Design review of the part built by this model. Coordinates are the model's own, in mm. Face numbers are marked on the shaded views. A direction names the side the tool comes from. Coordinates: 2 decimals unless noted, no trailing zeros. Loops run counter-clockwise (first coordinate to the right, second up) from the corner with the lowest first, then second, coordinate; pieces in that order, holes last. Notation, with made-up numbers: (34, 38) -> (65, 38) arc R23 ccw to (65, 71) -> close; hole circle Ø6 at (52.25, 23.25). An arc over 180 degrees is marked (long way). Answer in a Markdown table with one row per item.
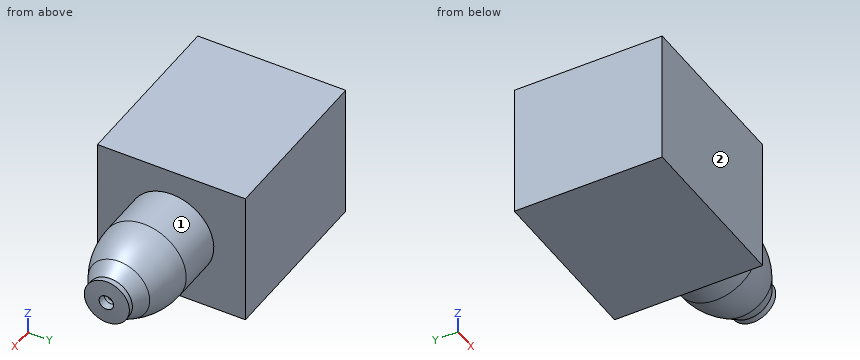
```python
from build123d import *

# Parameters (mm, degrees)
SKETCH1_W           = 52.054588137
SKETCH1_H           = 19.540614726
BOSS_EXTRUDE1_DEPTH = 8.89
SKETCH3_W           = 29.304045921
SKETCH3_H           = 19.540614726
CUT_EXTRUDE1_DEPTH  = 70.835641623


with BuildPart() as part:
    # Model → Revolve1 (revolve)
    with BuildSketch(Plane.XY, mode=Mode.PRIVATE) as revolve1_sk:
        with BuildLine():
            add(Edge.make_bspline(
                [(65.953268304, 2.93538911), (66.613970922, 2.97512211), (66.714344102, 2.980580933)],
                knots=[0.156174428, 0.156174428, 0.156174428, 1, 1, 1], degree=2))
            Line((66.714344102, 2.980580933), (66.8238694, 0.9515348))
            add(Edge.make_bspline(
                [(65.809518177, 0.891062762), (66.723641, 0.9461246), (66.8238694, 0.9515348)],
                knots=[0, 0, 0, 1, 1, 1], degree=2))
            ThreePointArc((65.809518177, 0.891062762), (65.799300412, 0.890601575), (65.7890734, 0.8904478))
            ThreePointArc((65.7890734, 0.8904478), (65.443371388, 0.935970102), (65.1212312, 1.0694162))
            Line((65.1212312, 1.0694162), (62.962634994, 2.315661898))
            ThreePointArc((62.962634994, 2.315661898), (60.719228535, 3.244897306), (58.3117616, 3.561842))
            Line((58.3117616, 3.561842), (0, 3.561842))
            Line((0, 3.561842), (0, 5.593842))
            Line((0, 5.593842), (58.3117616, 5.593842))
            ThreePointArc((58.3117616, 5.593842), (61.245141878, 5.207660449), (63.978622519, 4.075432721))
            Line((63.978622519, 4.075432721), (65.953268304, 2.93538911))
        make_face()
    revolve(revolve1_sk.sketch.rotate(Axis((0, 0, 0), (1, 0, 0)), 90), axis=Axis((0, 0, 0), (1, 0, 0)))

    # Sketch1 → Boss-Extrude1 (add, symmetric)
    with BuildSketch(Plane.XY):
        with Locations((26.027294069, 0)):
            Rectangle(SKETCH1_W, SKETCH1_H)
    extrude(amount=BOSS_EXTRUDE1_DEPTH, both=True)

    # Sketch3 → Cut-Extrude1 (cut, through all)
    with BuildSketch(Plane.XY.offset(8.89)):
        with Locations((14.652022961, 0)):
            Rectangle(SKETCH3_W, SKETCH3_H)
    extrude(amount=-CUT_EXTRUDE1_DEPTH, mode=Mode.SUBTRACT)


solid = part.part
```
(1) For pin 1 (5.5 mm diameter, centred on y = 3, z = -3, fed in from +X); pin 2 (2 mm diameter, centred on x = 53.5, z = -6, fed in from +Y); pin 3 (5 mm diameter, centred on x = 58, y = -5.5, fed in from -Z), all flat-tipped, find the tip position at first contact; note any pin that passes through.
Evaluation:
| item | result |
|---|---|
| pin 1 | stops at x = 66.79 |
| pin 2 | stops at y = 2.51 |
| pin 3 | stops at z = -4.72 |
(2) To check wall thickness, follow probe 1 along Y at (x, z) = (53.75, 0); probe 2 along Z at (x, y) = (54.5, 0.25); probe 3 along X at (y, z) = (6.5, -4.75). State the ranges of each line that lie inside material, in increasing order.
Evaluation:
| item | result |
|---|---|
| probe 1 | y = -5.59 to -3.56, 3.56 to 5.59 |
| probe 2 | z = -5.59 to -3.55, 3.55 to 5.59 |
| probe 3 | x = 29.3 to 52.05 |
(3) Take a section at A-A on y = 6.5. Give the boundary of the cut face in (x, z).
Evaluation:
| item | result |
|---|---|
| outline | (29.3, -8.89) -> (52.05, -8.89) -> (52.05, 8.89) -> (29.3, 8.89) -> close |
(4) Tool access review of the marked faces 1 and 2: name each direction out of +Z, -Z, +X, -X, +Y, -Y from which nothing blocks a thin tool from reaching the whole face with its end or side.
Evaluation:
| item | result |
|---|---|
| face 1 | +X |
| face 2 | +Z, -Z, +X, -X, -Y |
